For this review, take the finished solid that the model builds, in its own axes (mm). A direction names the side the tool comes from. Coordinates: 2 decimals unless noted, no trailing zeros. Write each loop counter-clockwise with the first axis right and the second up, starting at its lowest first coordinate (ties: lowest second). Pieces come first, ordered by that corner, then holes. Notation, with made-up numbers: (89.25, 9) -> (147.25, 9) arc R13 ccw to (147.25, 20) -> close; hole circle Ø4 at (72, -5). An arc over 180 degrees is marked (long way). One line per item, written item: value. Start each with the question number.
1) Machinability: for faces 1 (the flat face through (25.4, -42, 75)), 2 (the flat face through (190.5, -41, 6)), which of the approach directions +Z, -Z, +X, -X, +Y, -Y give a long, thin tool a straight path to every point of the face, cutting with its end or side? Answer none if there is none.
2) Add section C-C (z = 47). State the section outline as (x, y) points, and give its area (3 significant figures).
3) For probe 1 along Z at (x, y) = (39, -68); probe 2 along X at (y, z) = (-49, 52.5), list the stretches that pass through material, from the lowest coordinate up. Write a range as from..to.
4) Add section B-B (x = 59.5). State the section outline as (y, z) points, and give its area (3 significant figures).
5) Add section A-A (y = -76.5). State the section outline as (x, z) points, and give its area (3 significant figures).
6) For pin 1 Ø1 at (x, y) = (166.5, -52.5) entering from -Z; pin 2 Ø25 at (x, y) = (87, -48.5) entering from +Z; pin 3 Ø10 at (y, z) = (-69.5, 40.5) entering from +X, all flat-tipped, find the tip position at first contact; note any pin that passes through.
from build123d import *

# Parameters (mm, degrees)
F1_DEPTH = 82.55
F2_W     = 25.4
F2_H     = 82.55
F3_DEPTH = 127


with BuildPart() as f1:
    # F0 (on Front) → F1 (new body)
    with BuildSketch(Plane.XZ):
        Polygon((0, 12.7), (0, 0), (190.5, 0), (190.5, 12.7), (38.1, 12.7), align=None)
    extrude(amount=F1_DEPTH)

    # F2 (on face) → F3 (join)
    with BuildSketch(Plane.XY.offset(12.7)):
        with Locations((12.7, -41.275)):
            Rectangle(F2_W, F2_H)
    extrude(amount=F3_DEPTH)


solid = f1.part
Numbers:
1. face 1: +Z, +X, +Y, -Y
1. face 2: +Z, -Z, +X, +Y, -Y
2. outline: (0, -82.55) -> (25.4, -82.55) -> (25.4, 0) -> (0, 0) -> close
2. area: 2,100 mm²
3. probe 1: 0..12.7
3. probe 2: 0..25.4
4. outline: (-82.55, 0) -> (0, 0) -> (0, 12.7) -> (-82.55, 12.7) -> close
4. area: 1,050 mm²
5. outline: (0, 0) -> (190.5, 0) -> (190.5, 12.7) -> (25.4, 12.7) -> (25.4, 139.7) -> (0, 139.7) -> close
5. area: 5,650 mm²
6. pin 1: z = 0
6. pin 2: z = 12.7
6. pin 3: x = 25.4
